Input: part model. Units: mm. Frame: model coordinates. A direction names the side the tool comes from. Coordinates: 2 decimals unless noted, no trailing zeros. Order: outer loops, then holes, each group sorted by start corner. A loop starts at its lowest first (then second) coordinate and runs counter-clockwise, first axis right, second up. Notation, with made-up numbers: (18, 30.5) -> (35, 30.5) arc R34 cw to (35, 65.5) -> close; hole circle Ø9 at (72.25, 15). An arc over 180 degrees is marked (long way). One line per question, with ' | ' between items.
```python
from build123d import *

# Parameters (mm, degrees)
SKETCH1_R            = 2.413
EXTRUDE1_DEPTH       = 25.4
SKETCH6_R            = 3.9624
EXTRUDE2_DEPTH       = 4.826
CUT_EXTRUDE1_DEPTH   = 2.9765625
CHAMFER1_SIZE        = 0.39624
SKETCH10_R           = 2.413
PARTIAL_THREAD_DEPTH = 3.175
CHAMFER2_SIZE        = 0.09652


with BuildPart() as part:
    # Sketch1 → Extrude1 (new body)
    with BuildSketch(Plane.XY):
        Circle(SKETCH1_R)
    extrude(amount=-EXTRUDE1_DEPTH)

    # Sketch4 → Cut-Revolve1 (revolve, cut)
    with BuildSketch(Plane(origin=(0, 0, 0), x_dir=(0, 0, -1), z_dir=(1, 0, 0)), mode=Mode.PRIVATE) as cut_revolve1_sk:
        Polygon((0.659180743, 2.413), (0, 1.471592336), (0, 2.413), align=None)
    revolve(cut_revolve1_sk.sketch.rotate(Axis((0, 0, 0), (0, 0, -1)), 90), axis=Axis((0, 0, 0), (0, 0, -1)), mode=Mode.SUBTRACT)

    # Sketch6 → Extrude2 (add)
    with BuildSketch(Plane(origin=(0, 0, -25.4), x_dir=(-1, 0, 0), z_dir=(0, 0, -1))):
        Circle(SKETCH6_R)
    extrude(amount=EXTRUDE2_DEPTH)

    # Sketch7 → Cut-Extrude1 (cut)
    with BuildSketch(Plane(origin=(0, 0, -30.226), x_dir=(-1, 0, 0), z_dir=(0, 0, -1))):
        Polygon((0, 2.291358881), (-1.984375, 1.14567944), (-1.984375, -1.14567944), (0, -2.291358881), (1.984375, -1.14567944), (1.984375, 1.14567944), align=None)
    extrude(amount=-CUT_EXTRUDE1_DEPTH, mode=Mode.SUBTRACT)

    # Cut-Extrude2 cone 1 section (through the dimple's axis) → Cut-Extrude2 (revolve, cut)
    with BuildSketch(Plane(origin=(0, 0, -30.226), x_dir=(0, 1, 0), z_dir=(1, 0, 0))):
        Polygon((0, 0), (2.291358881, 0), (0, 2.291358881), align=None)
    revolve(axis=Axis((0, 0, -30.226), (0, 0, 1)), mode=Mode.SUBTRACT)

    # Chamfer1
    chamfer1_edges = [part.edges().sort_by_distance(p)[0] for p in [
        (3.9624, 0, -25.4),
        (3.9624, 0, -30.226),
    ]]
    chamfer(chamfer1_edges, length=CHAMFER1_SIZE)


with BuildPart() as body_2:
    # Sketch10 → partial thread (new body)
    with BuildSketch(Plane.XY.offset(-25.4)):
        Circle(SKETCH10_R)
    extrude(amount=PARTIAL_THREAD_DEPTH)

    # Chamfer2
    chamfer2_edges = [body_2.edges().sort_by_distance(p)[0] for p in [
        (-2.413, 0, -22.225),
    ]]
    chamfer(chamfer2_edges, length=CHAMFER2_SIZE)


with BuildPart() as part_1:
    add(part.part)

    # Combine1: union body 2
    add(body_2.part)


solid = part_1.part
```
1. Pin query (flat end, axial travel): pin 1 Ø1.1 at (y, z) = (-0.5, -28.5) entering from +X; pin 2 Ø2 at (x, y) = (0.5, 2.5) entering from +Z; pin 3 Ø2 at (x, z) = (3, -3) entering from -Y; pin 4 Ø1.5 at (x, z) = (2, -17) entering from +Y. Return the tip coordinate at first contact, or that it passes through.
Recorded:
pin 1: stops at x = 3.96 | pin 2: stops at z = -0.05 | pin 3: stops at y = -1.35 | pin 4: stops at y = 2.06
2. Cut plane B-B, the plane z = -22. Return loops of the section in (x, y).
Recorded:
outline: circle Ø4.83 at (0, 0)
3. Cut plane C-C, the plane z = -26.5. Return loops of the section in (x, y), and give its area (3 significant figures).
Recorded:
outline: circle Ø7.92 at (0, 0) | area: 49.3 mm^2
4. Access query for faces 4 (the face through (-1.984, 0, -29)), 5 (the face through (0, 0, 0)), 6 (the face through (-1.915, -1.468, -12.856)). Directions: +Z, -Z, +X, -X, +Y, -Y. A direction counts if a zero-diameter tool reaches every point of the face in a straight line with its end or side. Return the directions, or none.
Recorded:
face 4: -Z | face 5: +Z, +X, -X, +Y, -Y | face 6: +Z
5. Cut plane A-A, the plane y = 0. Return loops of the section in (x, z).
Recorded:
outline: (-3.96, -29.83) -> (-3.57, -30.23) -> (-2.29, -30.23) -> (-1.98, -29.92) -> (-1.98, -27.25) -> (1.98, -27.25) -> (1.98, -29.92) -> (2.29, -30.23) -> (3.57, -30.23) -> (3.96, -29.83) -> (3.96, -25.8) -> (3.57, -25.4) -> (2.41, -25.4) -> (2.41, -0.66) -> (1.47, 0) -> (-1.47, 0) -> (-2.41, -0.66) -> (-2.41, -25.4) -> (-3.57, -25.4) -> (-3.96, -25.8) -> close
6. Ray query, line 1 (Z direction, x = 0.25, y = -3.5); line 2 (Y direction, x = -0.75, z = -14). Return the intervals inside material, ascending. Write a range as [from, to].
Recorded:
line 1: z = [-30.23, -25.4] | line 2: y = [-2.29, 2.29]
7. Mould query, pull axis X, two halves, no side actions, for faces 1 (the face through (-2.33, -0.74, -30.226)), 2 (the face through (0.52, 3.93, -27.78)), 3 (the face through (0, 0, -27.249)). Classes: released by +X, released by -X, zero draft, split by the parting line, or undercut.
Recorded:
face 1: zero draft | face 2: split by the parting line | face 3: undercut
